The model under review builds one solid part; all positions refer to its coordinate system, in mm. Face numbers are marked on the shaded views. A direction names the side the tool comes from. Coordinates: 2 decimals unless noted, no trailing zeros. Write each loop counter-clockwise with the first axis right and the second up, starting at its lowest first coordinate (ties: lowest second). Pieces come first, ordered by that corner, then holes.
1) Add section C-C, the plane x = 100. State the section outline as (y, z) points (3 decimals), then the cut area to 3 significant figures.
2) Add section A-A, the plane x = 64.5. State the section outline as (y, z) points (3 decimals), then the cut area to 3 significant figures.
3) Mouldability with a two-part tool opening along X and no side actions: class the marked faces 6, 7 and 8 as released by +X, released by -X, zero draft, split by the parting line, or undercut.
4) Add section B-B, the plane y = -38.5. State the section outline as (x, z) points (3 decimals), then the cut area to 3 significant figures.
5) For line 1 (Z direction, x = 5.5, y = -30) (3 decimals); line 2 (X direction, y = 23.5, z = 5) (3 decimals); line 3 (Y direction, x = 86, z = 53.5), list the stretches that pass through material, from the lowest coordinate up.
6) Machinability: for the marked faces 1, 2, 3, 4 and 5, which of the approach directions +Z, -Z, +X, -X, +Y, -Y give a long, thin tool a straight path to every point of the face, cutting with its end or side? Answer none if there is none.
7) For P1, Ø3, axis at x = 75.5, z = 46.5, coming from the -Y side; P2, Ø4, axis at y = -19.5, z = 21.5, coming from the -X side (3 decimals); P3, Ø8, axis at x = 14, z = 22.5, coming from the -Y side, all flat-tipped, find the tip position at first contact; note any pin that passes through.
from build123d import *

# Parameters (mm, degrees)
F1_DEPTH = 63.5
F0_W     = 25.4
F0_H     = 19.05
F2_DEPTH = 25.4
F3_DEPTH = 12.7


with BuildPart() as f1:
    # F0 (on Front) → F1 (new body, symmetric)
    with BuildSketch(Plane.XZ):
        Polygon((-41.275, -9.525), (41.275, -9.525), (41.275, 9.525), (22.225, 9.525), (-41.275, 9.525), align=None)
    extrude(amount=F1_DEPTH, both=True)

    # F0 (on Front) → F2 (join, symmetric)
    with BuildSketch(Plane.XZ):
        with BuildLine():
            Line((22.225, 9.525), (41.275, 9.525))
            Line((41.275, 9.525), (41.275, 27.0002))
            ThreePointArc((41.275, 27.0002), (45.9246798487, 38.2255201513), (57.15, 42.8752))
            Line((57.15, 42.8752), (60.325, 42.8752))
            Line((60.325, 42.8752), (60.325, 61.9252))
            Line((60.325, 61.9252), (57.15, 61.9252))
            add(Edge.make_bspline(
                [(55.7747590851, 61.8981130812), (56.2330882006, 61.9086209195), (56.6915145362, 61.9176497894), (57.15, 61.9252)],
                knots=[110.4504448216, 110.4504448216, 110.4504448216, 110.4504448216, 111.5045361635, 111.5045361635, 111.5045361635, 111.5045361635], degree=3))
            ThreePointArc((55.7747590851, 61.8981130812), (31.9727690765, 51.2048001418), (22.225, 27.0002))
            Line((22.225, 27.0002), (22.225, 9.525))
        make_face()
        with Locations((73.025, 52.4002)):
            Rectangle(F0_W, F0_H)
    extrude(amount=F2_DEPTH, both=True)

    # F0 (on Front) → F3 (join, symmetric)
    with BuildSketch(Plane.XZ):
        with BuildLine():
            add(Edge.make_bspline(
                [(-41.275, 9.525), (-39.2076677015, 43.4578572164), (7.7498368859, 60.7970743394), (55.7747590851, 61.8981130812)],
                knots=[0, 0, 0, 0, 110.4504448216, 110.4504448216, 110.4504448216, 110.4504448216], degree=3))
            Line((-41.275, 9.525), (22.225, 9.525))
            Line((22.225, 9.525), (22.225, 27.0002))
            ThreePointArc((22.225, 27.0002), (31.9727690765, 51.2048001418), (55.7747590851, 61.8981130812))
        make_face()
    extrude(amount=F3_DEPTH, both=True)

    # F0 (on Front) → F4 (revolve)
    with BuildSketch(Plane.XZ):
        Polygon((85.725, 61.9252), (85.725, 42.8752), (85.725, 38.1), (111.125, 38.1), (111.125, 66.675), (85.725, 66.675), align=None)
    revolve(axis=Axis((85.725, 0, 52.3875), (0, 0, 1)))


solid = f1.part
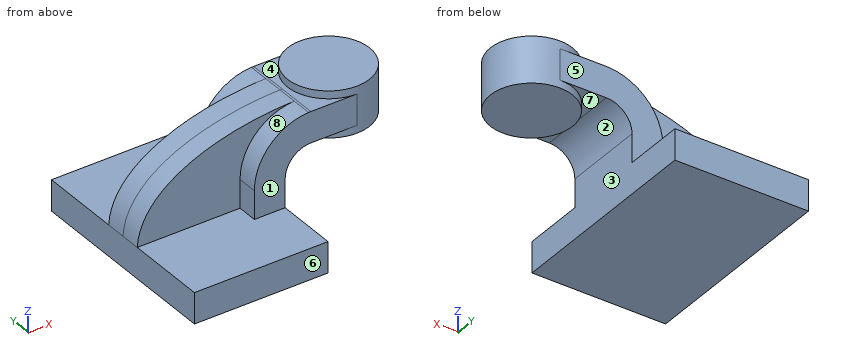
Geometry results:
1. outline: (-21.009, 38.1) - (21.009, 38.1) - (21.009, 66.675) - (-21.009, 66.675) - close
1. area: 1,200 mm2
2. outline: (-25.4, 42.875) - (-13.952, 42.875) - (-13.952, 38.1) - (13.952, 38.1) - (13.952, 42.875) - (25.4, 42.875) - (25.4, 61.925) - (13.952, 61.925) - (13.952, 66.675) - (-13.952, 66.675) - (-13.952, 61.925) - (-25.4, 61.925) - close
2. area: 1,230 mm2
3. face 6: zero draft
3. face 7: undercut
3. face 8: released by -X
4. outline: (-41.275, -9.525) - (41.275, -9.525) - (41.275, 9.525) - (-41.275, 9.525) - close
4. area: 1,570 mm2
5. line 1: z = -9.525 to 9.525
5. line 2: x = -41.275 to 41.275
5. line 3: y = -25.4 to 25.4
6. face 1: +Z, +X, -X, -Y
6. face 2: -Z, +Y, -Y
6. face 3: -Z, +X, +Y, -Y
6. face 4: +Z, -X
6. face 5: +Z, +X, -X, +Y
7. P1: stops at y = -25.4
7. P2: stops at x = 22.225
7. P3: stops at y = -12.7
